Read the model definition and answer for the solid it produces. Units are mm, in the model's axes. A direction names the side the tool comes from. Coordinates: 2 decimals unless noted, no trailing zeros. Loops run counter-clockwise (first coordinate to the right, second up) from the corner with the lowest first, then second, coordinate; pieces in that order, holes last. Notation, with made-up numbers: (-11.75, 48.25) - (41.25, 48.25) arc R19 cw to (41.25, 74.25) - close; hole circle Ø10 at (83.25, 77.25). An arc over 180 degrees is marked (long way). Use one line per item in the form item = value. Start each with the question number.
1) Consider line 1 (X direction, y = -97.5, z = 59) (3 decimals); line 2 (X direction, y = 185.5, z = 119.5); line 3 (Y direction, x = 160.5, z = 145). Determine where each line is inside the solid, lowest interval first.
2) Which of the six approach directions +Z, -Z, +X, -X, +Y, -Y give full straight-line access (tool end or side, diameter ignored) to faces 4 (the face through (91.04, -160.82, 3.62)), 5 (the face through (180.975, 1, 88)), 6 (the face through (-184.597, 1.565, 173.981)), 7 (the face through (-66, 190, 0))?
3) A cutting plane is placed at A-A (y = 0). Give the vertices of the cut face in (x, z) (3 decimals).
4) A cutting plane is placed at B-B (z = 19.5). Give the vertices of the cut face in (x, y) (3 decimals), and give its area (3 significant figures).
5) The mould has two halves that part along X. Classify faces 1 (the face through (-66, 190, 177.8)), 2 (the face through (-221.722, -170.011, 87.655)), 3 (the face through (-90.94, 160.65, 173.98)): released by +X, released by -X, zero draft, split by the parting line, or undercut.
6) A cutting plane is placed at C-C (x = 222). Give the vertices of the cut face in (y, z).
7) Each of these flat-tipped pins is pushed along its axis until it touches: P1, Ø3, axis at y = -9, z = 75.5, coming from the -X side; P2, Ø4, axis at x = -125, y = -146, coming from the +Z side; P3, Ø5, axis at x = -123, z = 111.5, coming from the -Y side. Where does it stop, or does it pass through?
from build123d import *

# Parameters (mm, degrees)
F0_R     = 279.4
F1_DEPTH = 177.8
F2_R     = 12.7
F3_R     = 12.7


with BuildPart() as f1:
    # F0 (on Top) → F1 (new body)
    with BuildSketch(Plane.XY):
        Circle(F0_R)
        Polygon((0, 208.97193), (180.975, 104.485965), (180.975, -104.485965), (0, -208.97193), (-180.975, -104.485965), (-180.975, 104.485965), align=None, mode=Mode.SUBTRACT)
    extrude(amount=F1_DEPTH)

    # F2
    f2_edges = [f1.edges().sort_by_distance(p)[0] for p in [
        (-90.4875, 156.728947, 177.8),
        (90.4875, 156.728947, 177.8),
        (-180.975, 0, 177.8),
        (-90.4875, -156.728947, 177.8),
        (90.4875, -156.728947, 177.8),
        (180.975, 0, 177.8),
    ]]
    fillet(f2_edges, radius=F2_R)

    # F3
    f3_edges = [f1.edges().sort_by_distance(p)[0] for p in [
        (-180.975, 0, 0),
        (-90.4875, -156.728947, 0),
        (90.4875, -156.728947, 0),
        (180.975, 0, 0),
        (90.4875, 156.728947, 0),
        (-90.4875, 156.728947, 0),
    ]]
    fillet(f3_edges, radius=F3_R)


solid = f1.part
Found:
q1.line_1 = -261.836 to -180.975, 180.975 to 261.836
q1.line_2 = -208.94 to -40.65, 40.65 to 208.94
q1.line_3 = -228.7 to -116.31, 116.31 to 228.7
q2.face_4 = -Z
q2.face_5 = +Z, -Z
q2.face_6 = +Z
q2.face_7 = -Z, +X, -X, +Y, -Y
q3.outline = (-279.4, 0) - (-193.675, 0) arc R12.7 ccw to (-180.975, 12.7) - (-180.975, 165.1) arc R12.7 ccw to (-193.675, 177.8) - (-279.4, 177.8) - close; (180.975, 12.7) arc R12.7 ccw to (193.675, 0) - (279.4, 0) - (279.4, 177.8) - (193.675, 177.8) arc R12.7 ccw to (180.975, 165.1) - close
q4.outline = circle Ø558.8 at (0, 0); hole (-180.975, -104.486) - (0, -208.972) - (180.975, -104.486) - (180.975, 104.486) - (0, 208.972) - (-180.975, 104.486) - close
q4.area = 132,000 mm^2
q5.face_1 = zero draft
q5.face_2 = split by the parting line
q5.face_3 = undercut
q6.outline = (-169.65, 0) - (169.65, 0) - (169.65, 177.8) - (-169.65, 177.8) - close
q7.P1 = -279.3
q7.P2 = 177.5
q7.P3 = -252.08
